```python
from build123d import *

# Parameters (mm, degrees)
SKETCH_1_R          = 3
EXTRUDE_1_DEPTH     = 120
CUT_EXTRUDE_1_DEPTH = 6


with BuildPart() as part:
    # Эскиз1 → Бобышка-Вытянуть1 (new body)
    with BuildSketch(Plane(origin=(0, 0, 0), x_dir=(0, 0, -1), z_dir=(1, 0, 0))):
        with BuildLine():
            Line((-15, 2.5), (-7.071067812, 2.5))
            ThreePointArc((-7.071067812, 2.5), (0, 7.5), (7.071067812, 2.5))
            Line((7.071067812, 2.5), (15, 2.5))
            Line((15, 2.5), (15, -2.5))
            Line((15, -2.5), (7.071067812, -2.5))
            ThreePointArc((7.071067812, -2.5), (0, -7.5), (-7.071067812, -2.5))
            Line((-7.071067812, -2.5), (-15, -2.5))
            Line((-15, -2.5), (-15, 2.5))
        make_face()
        Circle(SKETCH_1_R, mode=Mode.SUBTRACT)
    extrude(amount=EXTRUDE_1_DEPTH)

    # Эскиз2 → Вырез-Вытянуть1 (cut)
    with BuildSketch(Plane.ZY):
        Polygon((1.688931143, 3.671627014), (4.024187839, 0.373156232), (2.335256696, -3.298470782), (-1.688931143, -3.671627014), (-4.024187839, -0.373156232), (-2.335256696, 3.298470782), align=None)
    extrude(amount=-CUT_EXTRUDE_1_DEPTH, mode=Mode.SUBTRACT)


solid = part.part
```
Input: part model. Units: mm. Frame: model coordinates. A direction names the side the tool comes from. Give positions to 0.01 mm unless a question says otherwise; leave off trailing zeros. Write each loop counter-clockwise with the first axis right and the second up, starting at its lowest first coordinate (ties: lowest second). Pieces come first, ordered by that corner, then holes. Notation, with made-up numbers: (80.5, 43) - (127.5, 43) arc R23 ccw to (127.5, 63) - close; hole circle Ø2 at (81, 67). An arc over 180 degrees is marked (long way). Write item = value, one per line. Start each with the question number.
1) Cut plane D-D (z = 9.5). Return loops of the section in (x, y).
2) Pin query (flat end, axial travel): pin 1 (4 mm diameter, centred on x = 75.5, z = 12, fed in from -Y); pin 2 (2 mm diameter, centred on x = 60, y = -5, fed in from +Z); pin 3 (10 mm diameter, centred on x = 27, z = 9.5, fed in from -Y); pin 4 (3.5 mm diameter, centred on y = 0, z = 0, fed in from -X). Return the tip coordinate at first contact, or that it passes through.
3) Cut plane A-A (x = 15). Return loops of the section in (y, z), and give its area (3 significant figures).
4) Material intervals for L1, parallel to Z at x = 93.5, y = 0; L2, parallel to Y at x = 30.5, z = 0; L3, parallel to Y at x = 15, z = 11, sorted ascending. Write a range as [from, to].
5) Cut plane B-B (y = 1.5). Return loops of the section in (x, z).
6) Cut plane C-C (z = 0). Return loops of the section in (x, y), and give its area (3 significant figures).
7) Reachability of faces 1 (the face through (59, -2.5, 11)), 2 (the face through (59, 2.5, -11)), 3 (the face through (2.958, 2.045, 2.84)), 4 (the face through (59, -2.5, -11)), 5 (the face through (59, 2.5, 11)) from +Z, -Z, +X, -X, +Y, -Y: full face, straight path, thin tool, end or side. Return the list, or none.
Answers follow:
q1.outline = (0, -2.5) - (120, -2.5) - (120, 2.5) - (0, 2.5) - close
q2.pin_1 = -2.5
q2.pin_2 = 6.34
q2.pin_3 = -6
q2.pin_4 = through
q3.outline = (-2.5, -15) - (2.5, -15) - (2.5, -7.07) arc R7.5 ccw to (2.5, 7.07) - (2.5, 15) - (-2.5, 15) - (-2.5, 7.07) arc R7.5 ccw to (-2.5, -7.07) - close; hole circle Ø6 at (0, 0)
q3.area = 225 mm^2
q4.L1 = [-15, -3], [3, 15]
q4.L2 = [-7.5, -3], [3, 7.5]
q4.L3 = [-2.5, 2.5]
q5.outline = (0, -15) - (120, -15) - (120, -2.6) - (6, -2.6) - (6, -3.16) - (0, -3.16) - close; (0, 3.23) - (6, 3.23) - (6, 2.6) - (120, 2.6) - (120, 15) - (0, 15) - close
q6.outline = (0, -7.5) - (120, -7.5) - (120, -3) - (6, -3) - (6, -3.52) - (0, -3.52) - close; (0, 3.52) - (6, 3.52) - (6, 3) - (120, 3) - (120, 7.5) - (0, 7.5) - close
q6.area = 1,070 mm^2
q7.face_1 = +Z, +X, -X, -Y
q7.face_2 = -Z, +X, -X, +Y
q7.face_3 = -X
q7.face_4 = -Z, +X, -X, -Y
q7.face_5 = +Z, +X, -X, +Y
